CAD build for the part. Positions are in the model's coordinates, mm. A direction names the side the tool comes from. Round coordinates to 2 decimals unless told otherwise and drop trailing zeros. Order: outer loops, then holes, each group sorted by start corner. A loop starts at its lowest first (then second) coordinate and runs counter-clockwise, first axis right, second up. Notation, with made-up numbers: M -13,-31.75 L 7,-31.75 A24 cw 7,5.25 Z; hole C 68,85.5 d1. An arc over 180 degrees is marked long. Answer as a JSON object with one key per item and string values. Group by question number.
```python
from build123d import *

# Parameters (mm, degrees)
SKETCH1_R           = 1.35255
BOSS_EXTRUDE1_DEPTH = 3.175


with BuildPart() as part:
    # Sketch1 → Boss-Extrude1 (new body)
    with BuildSketch(Plane.XY):
        Polygon((2.291358881, 3.96875), (-2.291358881, 3.96875), (-4.582717762, 0), (-2.291358881, -3.96875), (2.291358881, -3.96875), (4.582717762, 0), align=None)
        Circle(SKETCH1_R, mode=Mode.SUBTRACT)
    extrude(amount=BOSS_EXTRUDE1_DEPTH)

    # Sketch2 → Cut-Revolve2 (revolve, cut)
    with BuildSketch(Plane(origin=(0, 0, 0), x_dir=(0, 0, -1), z_dir=(1, 0, 0)), mode=Mode.PRIVATE) as cut_revolve2_sk:
        with BuildLine():
            Line((-3.175, 3.96875), (-3.175, 2.910416667))
            ThreePointArc((-3.175, 2.910416667), (-2.865021343, 3.658771343), (-2.116666667, 3.96875))
            Line((-2.116666667, 3.96875), (-2.116666667, 5.953125))
            Line((-2.116666667, 5.953125), (-3.175, 5.953125))
            Line((-3.175, 5.953125), (-3.175, 3.96875))
        make_face()
    revolve(cut_revolve2_sk.sketch.rotate(Axis((0, 0, -0.15875), (0, 0, 1)), 90), axis=Axis((0, 0, -0.15875), (0, 0, 1)), mode=Mode.SUBTRACT)


solid = part.part
```
Item 1: Flat gauge pins, fed straight in: pin 1 Ø2 at (x, y) = (0, 0) entering from -Z; pin 2 Ø0.6 at (x, y) = (4, 0) entering from +Z; pin 3 Ø0.9 at (x, y) = (-4, -0.5) entering from +Z. Where does each tip first touch, or does it go through?
Item 2: 3-axis set-ups, long thin cutter, end or side, ignore diameter. For faces 5 (the face through (4.13, -0.01, 2.117)), 6 (the face through (2.1, 3.6, 2.117)), 7 (the face through (-2.1, 3.6, 2.117)): which of +Z, -Z, +X, -X, +Y, -Y reach the whole face in a straight line?
Item 3: Cut at B-B, the plane z = 2.35. Give the cut face in (x, y), and give its area (3 significant figures).
Item 4: Two-plate mould, pull along X, no slides. Class faces 1 (the face through (-2.1, -3.6, 2.117)), 2 (the face through (1.29, 0.41, 1.57)), 3 (the face through (3.42, -2.01, 1.04)), 4 (the face through (-3.45, -1.96, 1.04)): +X half, -X half, draft (parallel to the pull), parting line (faces both ways), or undercut.
Item 5: Cut at A-A, the plane z = 1.9. Give the cut face in (x, y).
Item 6: Drill centre lines: line 1 (Y direction, x = 0, z = 1.9); line 2 (Z direction, x = -4, y = -0.75); line 3 (Y direction, x = -1, z = 1.1). Where is each one in solid material? Low to high. Write a range as [from, to].
Response values:
{
 "1": {"pin 1": "through", "pin 2": "z = 2.82", "pin 3": "z = 2.94"},
 "2": {"face 5": "+Z, +X", "face 6": "+Z, +X, +Y", "face 7": "+Z, -X, +Y"},
 "3": {"outline": "C 0,0 d7.89; hole C 0,0 d2.71", "area": "43.1 mm^2"},
 "4": {"face 1": "draft", "face 2": "undercut", "face 3": "+X half", "face 4": "-X half"},
 "5": {"outline": "M -4.58,0 L -2.29,-3.97 L 2.29,-3.97 L 4.58,0 L 2.29,3.97 L -2.29,3.97 Z; hole C 0,0 d2.71"},
 "6": {"line 1": "[-3.97, -1.35], [1.35, 3.97]", "line 2": "[0, 2.12]", "line 3": "[-3.97, -0.91], [0.91, 3.97]"}
}
